Verification items for the finished model (mm, model axes). Coordinates: 2 decimals unless noted, no trailing zeros. Loops run counter-clockwise (first coordinate to the right, second up) from the corner with the lowest first, then second, coordinate; pieces in that order, holes last. Notation, with made-up numbers: (24, 18) -> (36, 18) arc R22 cw to (36, 46) -> close; hole circle Ø5 at (31.5, 82). An arc over 180 degrees is marked (long way). Answer as a JSON object with one key per item and string values. Group by question number.
Q1. Gauge pin test, flat ends, axial feed: pin 1 Ø1.5 at (y, z) = (-41.5, 2.5) entering from -X; pin 2 Ø1 at (y, z) = (-5.5, 0.5) entering from -X; pin 3 Ø1.5 at (y, z) = (3.5, 1.5) entering from -X. Record the tip position at first contact, or that the pin passes through.
Q2. Cross-section at A-A on x = 32. Record the boundary of the cut face in (y, z).
Q3. Cross-section at B-B on y = -33. Record the boundary of the cut face in (x, z), and give its area (3 significant figures).
Q4. Cross-section at D-D on x = -27. Record the boundary of the cut face in (y, z).
Q5. Cross-section at C-C on z = 1.6. Record the boundary of the cut face in (x, y), and give its area (3 significant figures).
Q6. Scan lines: L1, parallel to Y at x = 10, z = 1; L2, parallel to X at y = -54, z = 2.15; L3, parallel to X at y = -23, z = 1.35. Record each from-to range of solid material in increasing order.
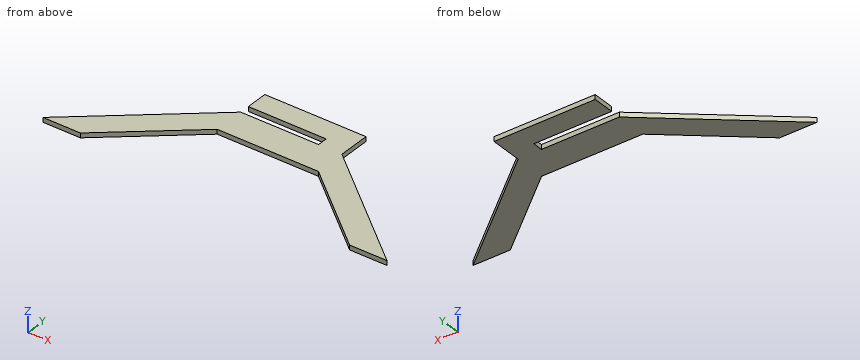
Autodesk Inventor part; units mm, degrees
ref_plane "YZ Plane" through (0, 0, 0) normal (1, 0, 0) x (0, 1, 0)
ref_plane "XZ Plane" through (0, 0, 0) normal (0, 1, 0) x (-1, 0, 0)
ref_plane "XY Plane" through (0, 0, 0) normal (0, 0, 1) x (1, 0, 0)
sketch "Sketch1" plane through (0, 0, 0) normal (0, 0, 1) x (1, 0, 0)
  line L0 (0, 20.5) -> (50, 20.5)
  line L1 (50, 20.5) -> (50, 6.5)
  line L2 (50, 6.5) -> (0, 6.5)
  line L3 (0, 6.5) -> (0, 20.5)
  line L4 (50, 20.5) -> (65, 20.5)
  line L5 (65, 20.5) -> (65, 0)
  line L6 (65, 0) -> (50, 0)
  line L7 (50, 0) -> (50, 20.5)
  line L8 (65, 0) -> (0, 0)
  line L9 (0, 0) -> (0, -20)
  line L10 (0, -20) -> (65, -20)
  line L11 (65, -20) -> (65, 0)
  line L12 (0, 0) -> (-78, -65)
  line L13 (-78, -65) -> (-54, -65)
  line L14 (-54, -65) -> (0, -20)
  line L15 (65, -20) -> (119, -65)
  line L16 (119, -65) -> (143, -65)
  line L17 (143, -65) -> (65, 0)
  point P0 (50, 6.5)
  point P1 (50, 0)
  dimension "d0" = 6.5
  dimension "d1" = 14
  dimension "d2" = 50
  dimension "d3" = 15
  dimension "d4" = 20
  dimension "d6" = 24
  dimension "d7" = 65
  dimension "d10" = 24
extrude "Extrusion1" add sketch "Sketch1" along normal blind 3
properties part number "Support_base"
Computed values:
{
 "1": {"pin 1": "stops at x = -50.7", "pin 2": "stops at x = -7.2", "pin 3": "stops at x = 50"},
 "2": {"outline": "(-20, 0) -> (0, 0) -> (0, 3) -> (-20, 3) -> close; (6.5, 0) -> (20.5, 0) -> (20.5, 3) -> (6.5, 3) -> close"},
 "3": {"outline": "(-39.6, 0) -> (-15.6, 0) -> (-15.6, 3) -> (-39.6, 3) -> close; (80.6, 0) -> (104.6, 0) -> (104.6, 3) -> (80.6, 3) -> close", "area": "144 mm²"},
 "4": {"outline": "(-42.5, 0) -> (-22.5, 0) -> (-22.5, 3) -> (-42.5, 3) -> close"},
 "5": {"outline": "(-78, -65) -> (-54, -65) -> (0, -20) -> (65, -20) -> (119, -65) -> (143, -65) -> (65, 0) -> (65, 20.5) -> (0, 20.5) -> (0, 6.5) -> (50, 6.5) -> (50, 0) -> (0, 0) -> close", "area": "4,950 mm²"},
 "6": {"L1": "y = -20 to 0, 6.5 to 20.5", "L2": "x = -64.8 to -40.8, 105.8 to 129.8", "L3": "x = -27.6 to -3.6, 68.6 to 92.6"}
}
